from build123d import *

# Parameters (mm, degrees)
ESQUISSE1_W               = 45
ESQUISSE1_H               = 20
BOSS_EXTRU_1_DEPTH        = 1
ENL_V_MAT_EXTRU_1_REACH   = 26.642
ESQUISSE2_R               = 0.75
SYM_TRIE2_COPY_1_REACH    = 26.642
SYM_TRIE2_COPY_1_SKETCH_R = 0.75
ESQUISSE3_R               = 7.5
BOSS_EXTRU_2_DEPTH        = 12
CONG_1_R                  = 0.5
BOSS_EXTRU_3_DEPTH        = 3
CONG_2_R                  = 0.1
ESQUISSE5_W               = 10
ESQUISSE5_H               = 2
BOSS_EXTRU_4_DEPTH        = 4
ESQUISSE6_W               = 10
ESQUISSE6_H               = 1
BOSS_EXTRU_5_DEPTH        = 6
ENL_V_MAT_EXTRU_2_REACH   = 33.611
ESQUISSE7_W               = 1.5
ESQUISSE7_H               = 2
ESQUISSE7_W_2             = 0.75
CHANFREIN1_SIZE           = 0.1
CONG_3_R                  = 0.3


with BuildPart() as part:
    # Esquisse1 → Boss.-Extru.1 (new body)
    with BuildSketch(Plane(origin=(0, 0, 0), x_dir=(1, 0, 0), z_dir=(0, 1, 0))):
        Rectangle(ESQUISSE1_W, ESQUISSE1_H)
    extrude(amount=BOSS_EXTRU_1_DEPTH)

    # Esquisse2 → Enlèv. mat.-Extru.1 (cut, up to next)
    with BuildSketch(Plane(origin=(0, 1, 0), x_dir=(1, 0, 0), z_dir=(0, 1, 0)), mode=Mode.PRIVATE) as enl_v_mat_extru_1_sk1:
        with Locations(Location((-21.5, 9, 0), (0, 0, 270))):
            Circle(ESQUISSE2_R)
    enl_v_mat_extru_1_tool1 = extrude(enl_v_mat_extru_1_sk1.sketch, amount=-ENL_V_MAT_EXTRU_1_REACH, mode=Mode.PRIVATE) & part.part
    enl_v_mat_extru_1 = enl_v_mat_extru_1_tool1.solids().sort_by_distance((-21.5, 1, -9))[0]
    add(enl_v_mat_extru_1, mode=Mode.SUBTRACT)

    # Symétrie1: Enlèv. mat.-Extru.1 across plane
    add(enl_v_mat_extru_1.mirror(Plane(origin=(0, 0, 0), x_dir=(0, 0, 1), z_dir=(1, 0, 0))), mode=Mode.SUBTRACT)

    # Symétrie2: Enlèv. mat.-Extru.1 across plane
    add(enl_v_mat_extru_1.mirror(Plane.XY), mode=Mode.SUBTRACT)

    # Symétrie2 copy 1 sketch → Symétrie2 copy 1 (cut, up to next)
    with BuildSketch(Plane(origin=(0, 1, 0), x_dir=(-1, 0, 0), z_dir=(0, 1, 0)), mode=Mode.PRIVATE) as sym_trie2_copy_1_sk1:
        with Locations(Location((-21.5, 9, 0), (0, 0, 270))):
            Circle(SYM_TRIE2_COPY_1_SKETCH_R)
    sym_trie2_copy_1_tool1 = extrude(sym_trie2_copy_1_sk1.sketch, amount=-SYM_TRIE2_COPY_1_REACH, mode=Mode.PRIVATE) & part.part
    add(sym_trie2_copy_1_tool1.solids().sort_by_distance((21.5, 1, 9))[0], mode=Mode.SUBTRACT)

    # Esquisse3 → Boss.-Extru.2 (add)
    with BuildSketch(Plane(origin=(0, 1, 0), x_dir=(1, 0, 0), z_dir=(0, 1, 0))):
        with Locations(Location((-12.5, 0, 0), (0, 0, 90))):
            Circle(ESQUISSE3_R)
        with Locations(Location((12.5, 0, 0), (0, 0, 90))):
            Circle(ESQUISSE3_R)
    extrude(amount=BOSS_EXTRU_2_DEPTH)

    # Congé1
    cong_1_edges = [part.edges().sort_by_distance(p)[0] for p in [
        (-12.5, 13, 7.5),
        (12.5, 13, 7.5),
    ]]
    fillet(cong_1_edges, radius=CONG_1_R)

    # Esquisse4 → Boss.-Extru.3 (add)
    with BuildSketch(Plane(origin=(0, 1, 0), x_dir=(1, 0, 0), z_dir=(0, 1, 0))):
        with BuildLine():
            Line((-3.5, 8.5), (3.5, 8.5))
            ThreePointArc((3.5, 8.5), (5, 7), (3.5, 5.5))
            Line((3.5, 5.5), (-3.5, 5.5))
            ThreePointArc((-3.5, 5.5), (-5, 7), (-3.5, 8.5))
        make_face()
    extrude(amount=BOSS_EXTRU_3_DEPTH)

    # Congé2
    cong_2_edges = [part.edges().sort_by_distance(p)[0] for p in [
        (-5, 4, -7),
        (0, 4, -5.5),
        (5, 4, -7),
        (0, 4, -8.5),
    ]]
    fillet(cong_2_edges, radius=CONG_2_R)

    # Esquisse5 → Boss.-Extru.4 (add)
    with BuildSketch(Plane.XZ):
        with Locations((0, 9)):
            Rectangle(ESQUISSE5_W, ESQUISSE5_H)
    extrude(amount=BOSS_EXTRU_4_DEPTH)

    # Esquisse6 → Boss.-Extru.5 (add)
    with BuildSketch(Plane.XY.offset(10)):
        with Locations((0, -3.5)):
            Rectangle(ESQUISSE6_W, ESQUISSE6_H)
    extrude(amount=BOSS_EXTRU_5_DEPTH)

    # Esquisse7 → Enlèv. mat.-Extru.2 (cut, up to next)
    with BuildSketch(Plane(origin=(0, 0, 8), x_dir=(-1, 0, 0), z_dir=(0, 0, -1)), mode=Mode.PRIVATE) as enl_v_mat_extru_2_sk1:
        with Locations((-2.5, -3)):
            Rectangle(ESQUISSE7_W, ESQUISSE7_H)
    enl_v_mat_extru_2_tool1 = extrude(enl_v_mat_extru_2_sk1.sketch, amount=-ENL_V_MAT_EXTRU_2_REACH, mode=Mode.PRIVATE) & part.part
    # Esquisse7 → Enlèv. mat.-Extru.2 (cut, up to next)
    with BuildSketch(Plane(origin=(0, 0, 8), x_dir=(-1, 0, 0), z_dir=(0, 0, -1)), mode=Mode.PRIVATE) as enl_v_mat_extru_2_sk2:
        with Locations((-4.625, -3)):
            Rectangle(ESQUISSE7_W_2, ESQUISSE7_H)
    enl_v_mat_extru_2_tool2 = extrude(enl_v_mat_extru_2_sk2.sketch, amount=-ENL_V_MAT_EXTRU_2_REACH, mode=Mode.PRIVATE) & part.part
    # Esquisse7 → Enlèv. mat.-Extru.2 (cut, up to next)
    with BuildSketch(Plane(origin=(0, 0, 8), x_dir=(-1, 0, 0), z_dir=(0, 0, -1)), mode=Mode.PRIVATE) as enl_v_mat_extru_2_sk3:
        with Locations((0, -3)):
            Rectangle(ESQUISSE7_W, ESQUISSE7_H)
    enl_v_mat_extru_2_tool3 = extrude(enl_v_mat_extru_2_sk3.sketch, amount=-ENL_V_MAT_EXTRU_2_REACH, mode=Mode.PRIVATE) & part.part
    # Esquisse7 → Enlèv. mat.-Extru.2 (cut, up to next)
    with BuildSketch(Plane(origin=(0, 0, 8), x_dir=(-1, 0, 0), z_dir=(0, 0, -1)), mode=Mode.PRIVATE) as enl_v_mat_extru_2_sk4:
        with Locations((2.5, -3)):
            Rectangle(ESQUISSE7_W, ESQUISSE7_H)
    enl_v_mat_extru_2_tool4 = extrude(enl_v_mat_extru_2_sk4.sketch, amount=-ENL_V_MAT_EXTRU_2_REACH, mode=Mode.PRIVATE) & part.part
    # Esquisse7 → Enlèv. mat.-Extru.2 (cut, up to next)
    with BuildSketch(Plane(origin=(0, 0, 8), x_dir=(-1, 0, 0), z_dir=(0, 0, -1)), mode=Mode.PRIVATE) as enl_v_mat_extru_2_sk5:
        with Locations((4.625, -3)):
            Rectangle(ESQUISSE7_W_2, ESQUISSE7_H)
    enl_v_mat_extru_2_tool5 = extrude(enl_v_mat_extru_2_sk5.sketch, amount=-ENL_V_MAT_EXTRU_2_REACH, mode=Mode.PRIVATE) & part.part
    add(enl_v_mat_extru_2_tool1.solids().sort_by_distance((2.5, -3, 8))[0], mode=Mode.SUBTRACT)
    add(enl_v_mat_extru_2_tool2.solids().sort_by_distance((4.625, -3, 8))[0], mode=Mode.SUBTRACT)
    add(enl_v_mat_extru_2_tool3.solids().sort_by_distance((0, -3, 8))[0], mode=Mode.SUBTRACT)
    add(enl_v_mat_extru_2_tool4.solids().sort_by_distance((-2.5, -3, 8))[0], mode=Mode.SUBTRACT)
    add(enl_v_mat_extru_2_tool5.solids().sort_by_distance((-4.625, -3, 8))[0], mode=Mode.SUBTRACT)

    # Chanfrein1
    chanfrein1_edges = [part.edges().sort_by_distance(p)[0] for p in [
        (-3.75, -3, 16),
        (-4.25, -3.5, 16),
        (-1.75, -3.5, 16),
        (-3.25, -3.5, 16),
        (0.75, -3.5, 16),
        (-0.75, -3.5, 16),
        (4.25, -3.5, 16),
        (3.25, -3.5, 16),
        (1.75, -3.5, 16),
        (-3.75, -4, 16),
        (-1.25, -4, 16),
        (1.25, -4, 16),
        (3.75, -4, 16),
        (3.75, -3, 16),
        (1.25, -3, 16),
        (-1.25, -3, 16),
    ]]
    chamfer(chanfrein1_edges, length=CHANFREIN1_SIZE)

    # Congé3
    cong_3_edges = [part.edges().sort_by_distance(p)[0] for p in [
        (3.75, -3, 10),
        (1.25, -3, 10),
        (-1.25, -3, 10),
        (-3.75, -3, 10),
        (-3.75, -4, 8),
        (-1.25, -4, 8),
        (1.25, -4, 8),
        (3.75, -4, 8),
    ]]
    fillet(cong_3_edges, radius=CONG_3_R)


solid = part.part
Check sheet for the modelled part. Datum: model origin and axes. Units: mm. A direction names the side the tool comes from. Round coordinates to 2 decimals unless told otherwise and drop trailing zeros. Order: outer loops, then holes, each group sorted by start corner. A loop starts at its lowest first (then second) coordinate and runs counter-clockwise, first axis right, second up.
(1) Access from +Z, -Z, +X, -X, +Y, -Y to the whole of each face (thin tool, end or side, straight path). Record for faces 1 (the flat face through (-1.75, -3.2, 11)), 2 (the flat face through (5, -1, 9)), 3 (the flat face through (-4.25, -3.2, 11)), 4 (the flat face through (0, 4, -7)).
(2) Cross-section at A-A, the plane z = -9. Enter the section's corners in (x, y), and give its area (3 significant figures).
(3) Draft check along Z on faces 5 (the flat face through (0, -1, 8)), 6 (the flat face through (-13, 13, 0)), 7 (the cylindrical face through (22.232, 0.507, 9.163)). Enter one of: pulls with the +Z half, pulls with the -Z half, needs draft (parallel to the pull), parting line crosses it, or undercut.
(4) Cross-section at D-D, the plane x = 12.5. Enter the section's corners in (y, z).
(5) Scan lines: probe 1 along X at (y, z) = (0.55, 9); probe 2 along Z at (x, y) = (21.5, 0.6); probe 3 along Y at (x, z) = (-16, 1.25). Record each from-to range of solid material in increasing order.
(6) Go/stop test with flat-tipped pins: P1, Ø1.1, axis at x = -4, z = 12.5, coming from the +Y side; P2, Ø1.6, axis at y = -3.5, z = 11.5, coming from the -X side; P3, Ø3, axis at x = 2.5, y = -1, coming from the +Z side. Record where each tip stops, or that it passes through.
(7) Cross-section at B-B, the plane z = 11.5. Enter the section's corners in (x, y).
(8) Cross-section at C-C, the plane x = -21.5. Enter the section's corners in (y, z).
Check sheet entries:
1. face 1: +Z, -Z, -Y
1. face 2: +Z, -Z, +X, -Y
1. face 3: +Z, -Z, -X, -Y
1. face 4: +Z, -Z, +Y
2. outline: (-22.5, 0) - (-22.25, 0) - (-22.25, 1) - (-22.5, 1) - close; (-20.75, 0) - (20.75, 0) - (20.75, 1) - (-20.75, 1) - close; (22.25, 0) - (22.5, 0) - (22.5, 1) - (22.25, 1) - close
2. area: 42.0 mm2
3. face 5: pulls with the -Z half
3. face 6: needs draft
3. face 7: undercut
4. outline: (0, -10) - (1, -10) - (1, -7.5) - (12.5, -7.5) arc R0.5 ccw to (13, -7) - (13, 7) arc R0.5 ccw to (12.5, 7.5) - (1, 7.5) - (1, 10) - (0, 10) - close
5. probe 1: x = -22.5 to -22.25, -20.75 to 20.75, 22.25 to 22.5
5. probe 2: z = -10 to -9.75, -8.25 to 8.25, 9.75 to 10
5. probe 3: y = 0 to 13
6. P1: stops at y = -3
6. P2: stops at x = -4.25
6. P3: stops at z = 10
7. outline: (-4.25, -4) - (-3.25, -4) - (-3.25, -3) - (-4.25, -3) - close; (-1.75, -4) - (-0.75, -4) - (-0.75, -3) - (-1.75, -3) - close; (0.75, -4) - (1.75, -4) - (1.75, -3) - (0.75, -3) - close; (3.25, -4) - (4.25, -4) - (4.25, -3) - (3.25, -3) - close
8. outline: (0, -10) - (1, -10) - (1, -9.75) - (0, -9.75) - close; (0, -8.25) - (1, -8.25) - (1, 8.25) - (0, 8.25) - close; (0, 9.75) - (1, 9.75) - (1, 10) - (0, 10) - close
